from build123d import *

# Parameters (mm, degrees)
BOSS_EXTRUDE1_DEPTH = 15
FILLET1_R           = 0.5


with BuildPart() as part:
    # Sketch1 → Boss-Extrude1 (new body)
    with BuildSketch(Plane.XY):
        with BuildLine():
            Line((0, 0), (20, 0))
            Line((20, 0), (20, 8.778684822))
            ThreePointArc((20, 8.778684822), (10, 7), (0, 8.778684822))
            Line((0, 8.778684822), (0, 0))
        make_face()
    extrude(amount=BOSS_EXTRUDE1_DEPTH)

    # Fillet1
    fillet1_edges = [part.edges().sort_by_distance(p)[0] for p in [
        (20, 4.389342411, 15),
        (10, 7, 15),
        (0, 4.389342411, 15),
        (10, 7, 0),
        (20, 4.389342411, 0),
        (0, 4.389342411, 0),
        (0, 8.778684822, 7.5),
        (20, 8.778684822, 7.5),
    ]]
    fillet(fillet1_edges, radius=FILLET1_R)


solid = part.part
Design review of the part built by this model. Coordinates are the model's own, in mm. Give positions to 0.01 mm unless a question says otherwise; leave off trailing zeros. Loops run counter-clockwise (first coordinate to the right, second up) from the corner with the lowest first, then second, coordinate; pieces in that order, holes last. Notation, with made-up numbers: (65, -29) - (96, -29) arc R19 cw to (96, -7) - close; hole circle Ø5 at (79.25, 34.5). An arc over 180 degrees is marked (long way). Write item = value, one per line.
1) To check wall thickness, follow line 1 (Y direction, x = 14, z = 8); line 2 (Y direction, x = 18, z = 13). State the ranges of each line that lie inside material, in increasing order.
Result sheet:
line_1 = 0 to 7.28
line_2 = 0 to 8.13
2) Take a section at B-B on z = 5.75. State the section outline as (x, y) points, and give its area (3 significant figures).
Result sheet:
outline = (0, 0) - (20, 0) - (20, 8.07) arc R0.5 ccw to (19.34, 8.54) arc R29 cw to (0.66, 8.54) arc R0.5 ccw to (0, 8.07) - close
area = 151 mm2
3) Take a section at A-A on x = 10. State the section outline as (y, z) points, and give its area (3 significant figures).
Result sheet:
outline = (0, 0) - (6.5, 0) arc R0.5 ccw to (7, 0.5) - (7, 14.5) arc R0.5 ccw to (6.5, 15) - (0, 15) - close
area = 105 mm2
4) Draft analysis for pull direction X (two halves, no side actions). For faces 1 (the face through (0, 4, 7)), 2 (the face through (20, 4, 7)), 3 (the face through (10, 7, 7)), state which applies: +X half, -X half, draft (parallel to the pull), parting line (faces both ways), or undercut.
Result sheet:
face_1 = -X half
face_2 = +X half
face_3 = undercut
